from build123d import *

# Parameters (mm, degrees)
F0_W     = 22.956962
F0_H     = 24
F0_R     = 0.5
F0_R_2   = 1.05
F1_DEPTH = 1.6
F2_W     = 19
F2_H     = 10.5
F3_DEPTH = 25


with BuildPart() as f1:
    # F0 (on Top) → F1 (new body)
    with BuildSketch(Plane.XY):
        with Locations((-0.186301, 0)):
            Rectangle(F0_W, F0_H)
        with Locations((2.54, -7.5)):
            Circle(F0_R, mode=Mode.SUBTRACT)
        with Locations((-2.5, 7.05)):
            Circle(F0_R, mode=Mode.SUBTRACT)
        with Locations((-5, 9.05)):
            Circle(F0_R_2, mode=Mode.SUBTRACT)
        with Locations((0, 7.05)):
            Circle(F0_R, mode=Mode.SUBTRACT)
        with Locations((2.5, 7.05)):
            Circle(F0_R, mode=Mode.SUBTRACT)
        with Locations((5, 9.05)):
            Circle(F0_R_2, mode=Mode.SUBTRACT)
    extrude(amount=-F1_DEPTH)

    # F2 (on face) → F3 (cut)
    with BuildSketch(Plane.XY):
        Rectangle(F2_W, F2_H)
    extrude(amount=-F3_DEPTH, mode=Mode.SUBTRACT)


solid = f1.part
Geometry: final body of the model. Coordinates: model frame, mm. A direction names the side the tool comes from. Round coordinates to 2 decimals unless told otherwise and drop trailing zeros. Loops run counter-clockwise (first coordinate to the right, second up) from the corner with the lowest first, then second, coordinate; pieces in that order, holes last.
Q1. Section A-A on y = 7.05. Return loops of the section in (x, z), plus the area to 3 significant figures.
Q2. Material intervals for L1, parallel to Y at x = 0, z = -0.8; L2, parallel to Y at x = -5, z = -1.2; L3, parallel to Y at x = 6.25, z = -0.65, sorted ascending.
Q3. Pull-direction query (Y, two-part tool) for faces 3 (the flat face through (0, -12, -1)), 4 (the flat face through (0, 6, -1.6)), 5 (the cylindrical face through (2.392, 6.562, -0.789)); classes: released by +Y, released by -Y, zero draft, split by the parting line, or undercut.
Q4. Section D-D on z = -0.75. Return loops of the section in (x, y), plus the area to 3 significant figures.
Q5. Section C-C on y = -1. Return loops of the section in (x, z), plus the area to 3 significant figures.
Q6. Access query for faces 1 (the flat face through (0, 5.25, -1)), 2 (the flat face through (-11.665, 0, -1)). Directions: +Z, -Z, +X, -X, +Y, -Y. A direction counts if a zero-diameter tool reaches every point of the face in a straight line with its end or side. Return the directions, or none.
Q7. Section B-B on x = 8. Return loops of the section in (y, z), plus the area to 3 significant figures.
Evaluation:
1. outline: (-11.66, -1.6) - (-3, -1.6) - (-3, 0) - (-11.66, 0) - close; (-2, -1.6) - (-0.5, -1.6) - (-0.5, 0) - (-2, 0) - close; (0.5, -1.6) - (2, -1.6) - (2, 0) - (0.5, 0) - close; (3, -1.6) - (11.29, -1.6) - (11.29, 0) - (3, 0) - close
1. area: 31.9 mm2
2. L1: y = -12 to -5.25, 5.25 to 6.55, 7.55 to 12
2. L2: y = -12 to -5.25, 5.25 to 8, 10.1 to 12
2. L3: y = -12 to -5.25, 5.25 to 12
3. face 3: released by -Y
3. face 4: zero draft
3. face 5: undercut
4. outline: (-11.66, -12) - (11.29, -12) - (11.29, 12) - (-11.66, 12) - close; hole (-9.5, -5.25) - (9.5, -5.25) - (9.5, 5.25) - (-9.5, 5.25) - close; hole circle Ø2.1 at (-5, 9.05); hole circle Ø1 at (-2.5, 7.05); hole circle Ø1 at (0, 7.05); hole circle Ø1 at (2.5, 7.05); hole circle Ø1 at (2.54, -7.5); hole circle Ø2.1 at (5, 9.05)
4. area: 341 mm2
5. outline: (-11.66, -1.6) - (-9.5, -1.6) - (-9.5, 0) - (-11.66, 0) - close; (9.5, -1.6) - (11.29, -1.6) - (11.29, 0) - (9.5, 0) - close
5. area: 6.33 mm2
6. face 1: +Z, -Z
6. face 2: +Z, -Z, -X, +Y, -Y
7. outline: (-12, -1.6) - (-5.25, -1.6) - (-5.25, 0) - (-12, 0) - close; (5.25, -1.6) - (12, -1.6) - (12, 0) - (5.25, 0) - close
7. area: 21.6 mm2
